```python
from build123d import *

# Parameters (mm, degrees)
SKETCH1_R                    = 11025
BOSS_EXTRUDE1_DEPTH          = 5000
BOSS_EXTRUDE2_DEPTH          = 8000
SKETCH4_R                    = 3000
CUT_EXTRUDE2_DEPTH           = 3000
SKETCH5_R                    = 1500
CUT_EXTRUDE3_DEPTH           = 3000
SKETCH6_R                    = 3000
CUT_EXTRUDE4_DEPTH           = 3000
SKETCH3_R                    = 2900
CUT_EXTRUDE1_DEPTH           = 12018
SCALE6_SCALE                 = 0.001
CORTAR_EXTRUIR1_DEPTH        = 10
CORTAR_EXTRUIR1_DEPTH_BACK   = 10
CROQUIS1_R                   = 12.5
CROQUIS2_W                   = 9
CROQUIS2_H                   = 0.876479878
CORTAR_EXTRUIR2_DEPTH        = 8
CROQUIS4_R                   = 2.9
CROQUIS4_R_2                 = 2.4
SALIENTE_EXTRUIR2_DEPTH      = 8.611616332
CROQUIS5_R                   = 3.5
CORTAR_EXTRUIR3_DEPTH        = 3
CROQUIS6_R                   = 1.591781054
CROQUIS6_R_2                 = 3
CROQUIS6_R_3                 = 1.5
CROQUIS6_R_4                 = 12.5
SALIENTE_EXTRUIR3_DEPTH      = 1
REDONDEO1_R                  = 2.5
TALADRO_DE_MARGEN_PARA_M51_D = 5.5
SALIENTE_EXTRUIR4_DEPTH      = 7
REDONDEO2_SIZE               = 2.5
REDONDEO2_SIZE_2             = 7.5


with BuildPart() as part:
    # Sketch1 → Boss-Extrude1 (new body)
    with BuildSketch(Plane.XY):
        Polygon((-21150, 17212.99935917), (-17091.781053823, 21271.218305346), (17091.781053823, 21271.218305346), (21150, 17212.99935917), (21150, -16970.562748477), (17091.781053823, -21028.781694654), (-17091.781053823, -21028.781694654), (-21150, -16970.562748477), align=None)
        with Locations((0, 121.218305346)):
            Circle(SKETCH1_R, mode=Mode.SUBTRACT)
    extrude(amount=BOSS_EXTRUDE1_DEPTH)

    # Sketch2 → Boss-Extrude2 (add)
    with BuildSketch(Plane.XY.offset(5000)):
        Polygon((0, -11028.781694654), (4500, -11028.781694654), (4500, -21028.781694654), (-4500, -21028.781694654), (-4500, -11028.781694654), align=None)
    extrude(amount=BOSS_EXTRUDE2_DEPTH)

    # Sketch4 → Cut-Extrude2 (cut)
    with BuildSketch(Plane.XY.offset(5000)):
        with Locations((-15500, 15500)):
            Circle(SKETCH4_R)
        with Locations((15500, 15500)):
            Circle(SKETCH4_R)
        with Locations((15500, -15500)):
            Circle(SKETCH4_R)
        with Locations((-15500, -15500)):
            Circle(SKETCH4_R)
    extrude(amount=-CUT_EXTRUDE2_DEPTH, mode=Mode.SUBTRACT)

    # Sketch5 → Cut-Extrude3 (cut)
    with BuildSketch(Plane.XY.offset(2000)):
        with Locations((-15500, 15500)):
            Circle(SKETCH5_R)
        with Locations((15500, -15500)):
            Circle(SKETCH5_R)
    extrude(amount=-CUT_EXTRUDE3_DEPTH, mode=Mode.SUBTRACT)

    # Sketch6 → Cut-Extrude4 (cut)
    with BuildSketch(Plane.XY.offset(2000)):
        with Locations((15500, 15500)):
            Circle(SKETCH6_R)
        with Locations((-15500, -15500)):
            Circle(SKETCH6_R)
    extrude(amount=-CUT_EXTRUDE4_DEPTH, mode=Mode.SUBTRACT)

    # Sketch3 → Cut-Extrude1 (cut)
    with BuildSketch(Plane.XZ.offset(21028.781694654)):
        with Locations(Location((0, 9000, 0), (0, 0, 270))):
            Circle(SKETCH3_R)
    extrude(amount=-CUT_EXTRUDE1_DEPTH, mode=Mode.SUBTRACT)


with BuildPart() as part_1:
    # Scale6: scaled about (0, -945.258123271, 2914.075668663)
    add(part.part.scale(SCALE6_SCALE).moved(Location((0, -944.312865148, 2911.161592994))))

    # Croquis1 → Cortar-Extruir1 (cut, two sides: drawn at the far end of the back side and taken through both)
    with BuildSketch(Plane.XY.offset(2916.161592994).offset(-CORTAR_EXTRUIR1_DEPTH_BACK)):
        with Locations(Location((0, -944.191646843, 0), (0, 0, 248.899803976))):
            Circle(CROQUIS1_R)
    extrude(amount=CORTAR_EXTRUIR1_DEPTH + CORTAR_EXTRUIR1_DEPTH_BACK, mode=Mode.SUBTRACT)

    # Croquis2 → Cortar-Extruir2 (cut)
    with BuildSketch(Plane.XY.offset(2924.161592994)):
        with Locations((0, -956.291790571)):
            Rectangle(CROQUIS2_W, CROQUIS2_H)
    extrude(amount=-CORTAR_EXTRUIR2_DEPTH, mode=Mode.SUBTRACT)

    # Croquis4 → Saliente-Extruir2 (add)
    with BuildSketch(Plane.XZ.offset(965.341646843)):
        with Locations((0, 2920.161592994)):
            Circle(CROQUIS4_R)
        with Locations(Location((0, 2920.161592994, 0), (0, 0, 270))):
            Circle(CROQUIS4_R_2, mode=Mode.SUBTRACT)
    extrude(amount=-SALIENTE_EXTRUIR2_DEPTH)

    # Croquis5 → Cortar-Extruir3 (cut)
    with BuildSketch(Plane.XY.offset(2916.161592994)):
        with Locations((-15.5, -928.812865148)):
            Circle(CROQUIS5_R)
        with Locations((15.5, -959.812865148)):
            Circle(CROQUIS5_R)
    extrude(amount=-CORTAR_EXTRUIR3_DEPTH, mode=Mode.SUBTRACT)

    # Croquis6 → Saliente-Extruir3 (add)
    with BuildSketch(Plane(origin=(0, 0, 2911.161592994), x_dir=(-1, 0, 0), z_dir=(0, 0, -1))):
        Polygon((17.091781054, -923.041646843), (-17.091781054, -923.041646843), (-21.15, -927.099865789), (-21.15, -961.283427896), (-17.091781054, -965.341646843), (17.091781054, -965.341646843), (21.15, -961.283427896), (21.15, -927.099865789), align=None)
        with Locations((15.5, -928.812865148)):
            Circle(CROQUIS6_R, mode=Mode.SUBTRACT)
        with Locations(Location((-15.5, -928.812865148, 0), (0, 0, 180))):
            Circle(CROQUIS6_R_2, mode=Mode.SUBTRACT)
        with Locations(Location((-15.5, -959.812865148, 0), (0, 0, 180))):
            Circle(CROQUIS6_R_3, mode=Mode.SUBTRACT)
        with Locations(Location((15.5, -959.812865148, 0), (0, 0, 180))):
            Circle(CROQUIS6_R_2, mode=Mode.SUBTRACT)
        with Locations((0, -944.191646843)):
            Circle(CROQUIS6_R_4, mode=Mode.SUBTRACT)
    extrude(amount=SALIENTE_EXTRUIR3_DEPTH)

    # Redondeo1
    redondeo1_edges = [part_1.edges().sort_by_distance(p)[0] for p in [
        (4.5, -961.035838676, 2924.161592994),
        (-4.5, -961.035838676, 2924.161592994),
    ]]
    fillet(redondeo1_edges, radius=REDONDEO1_R)

    # Taladro de margen para M51 (through all)
    with Locations(Plane(origin=(0, -956.73003051, 2920.161592994), x_dir=(0, 0, 1), z_dir=(0, 1, 0))):
        with Locations((0, 0)):
            Hole(TALADRO_DE_MARGEN_PARA_M51_D / 2)

    # Croquis8 → Saliente-Extruir4 (add)
    with BuildSketch(Plane.XZ.offset(965.341646843)):
        Polygon((-2.879289322, 2912.011592994), (-5.45, 2912.011592994), (-5.45, 2913.290882316), (-2.529289322, 2916.211592994), (2.429289322, 2916.211592994), (5.35, 2913.290882316), (5.35, 2912.011592994), (2.879289322, 2912.011592994), (2.879289322, 2910.161592994), (-2.879289322, 2910.161592994), align=None)
    extrude(amount=SALIENTE_EXTRUIR4_DEPTH)

    # Redondeo2
    # an asymmetric fillet: 7.5, 2.5 mm, written as the material it adds along each edge
    with BuildSketch(Plane(origin=(4.5, -956.73003051, 2916.161592994), x_dir=(0, 0, 1), z_dir=(0, -1, 0))) as redondeo2_piece_1:
        with BuildLine():
            Bezier((REDONDEO2_SIZE, 0), (0, 0), (0, -REDONDEO2_SIZE_2), weights=[1, 0.707106781, 1])
            Line((0, -REDONDEO2_SIZE_2), (0, 0))
            Line((0, 0), (REDONDEO2_SIZE, 0))
        make_face()
    extrude(amount=8.611616332)
    with BuildSketch(Plane(origin=(-4.5, -965.341646842, 2916.161592994), x_dir=(-1, 0, 0), z_dir=(0, 1, 0))) as redondeo2_piece_2:
        with BuildLine():
            Bezier((REDONDEO2_SIZE_2, 0), (0, 0), (0, REDONDEO2_SIZE), weights=[1, 0.707106781, 1])
            Line((0, REDONDEO2_SIZE), (0, 0))
            Line((0, 0), (REDONDEO2_SIZE_2, 0))
        make_face()
    extrude(amount=8.611616332)


solid = part_1.part
```
Can you work these out from the model? Positions are in its coordinate system, mm. A direction names the side the tool comes from. Round coordinates to 2 decimals unless told otherwise and drop trailing zeros. Loops run counter-clockwise (first coordinate to the right, second up) from the corner with the lowest first, then second, coordinate; pieces in that order, holes last. Notation, with made-up numbers: (45.5, 48) -> (59.5, 48) arc R12 ccw to (59.5, 61) -> close; hole circle Ø4 at (-27.75, 56.5). An arc over 180 degrees is marked (long way). Answer in a Markdown table with one row per item.
Item 1: Suppose I cut it at A-A, the plane x = 15.5. List the corners of the cut face in (y, z) for me, plus the area to 3 significant figures.
Answer block:
| item | result |
|---|---|
| outline | (-965.34, 2910.16) -> (-961.31, 2910.16) -> (-961.31, 2913.16) -> (-963.31, 2913.16) -> (-963.31, 2916.16) -> (-965.34, 2916.16) -> close; (-958.31, 2910.16) -> (-931.81, 2910.16) -> (-931.81, 2916.16) -> (-956.31, 2916.16) -> (-956.31, 2913.16) -> (-958.31, 2913.16) -> close; (-925.81, 2910.16) -> (-923.04, 2910.16) -> (-923.04, 2916.16) -> (-925.81, 2916.16) -> close |
| area | 188 mm² |
Item 2: Suppose I cut it at D-D, the plane x = -15.5. List the corners of the cut face in (y, z) for me.
Answer block:
| item | result |
|---|---|
| outline | (-965.34, 2910.16) -> (-962.81, 2910.16) -> (-962.81, 2916.16) -> (-965.34, 2916.16) -> close; (-956.81, 2910.16) -> (-930.4, 2910.16) -> (-930.4, 2911.16) -> (-930.31, 2911.16) -> (-930.31, 2913.16) -> (-932.31, 2913.16) -> (-932.31, 2916.16) -> (-956.81, 2916.16) -> close; (-927.31, 2911.16) -> (-927.22, 2911.16) -> (-927.22, 2910.16) -> (-923.04, 2910.16) -> (-923.04, 2916.16) -> (-925.31, 2916.16) -> (-925.31, 2913.16) -> (-927.31, 2913.16) -> close |
Item 3: Suppose I cut it at C-C, the plane z = 2920.25. List the corners of the cut face in (x, y) for me, plus the area to 3 significant figures.
Answer block:
| item | result |
|---|---|
| outline | (-4.5, -965.34) -> (-2.75, -965.34) -> (-2.75, -956.73) -> (-4.5, -956.73) -> close; (2.75, -965.34) -> (4.5, -965.34) -> (4.5, -956.73) -> (2.75, -956.73) -> close |
| area | 30.2 mm² |
Item 4: Suppose I cut it at B-B, the plane y = -946. List the corners of the cut face in (x, z) for me.
Answer block:
| item | result |
|---|---|
| outline | (-21.15, 2910.16) -> (-12.37, 2910.16) -> (-12.37, 2916.16) -> (-21.15, 2916.16) -> close; (12.37, 2910.16) -> (21.15, 2910.16) -> (21.15, 2916.16) -> (12.37, 2916.16) -> close |
Item 5: Will these pins go through, and if not, where does the flat tip stop? P1, Ø3.5, axis at x = -15.5, y = -928.5, coming from the -Z side; P2, Ø2, axis at y = -969, z = 2911.5, coming from the -X side; P3, Ø0.6, axis at y = -970, z = 2912.5, coming from the +X side; P4, Ø5, axis at x = 15.5, y = -928.81, coming from the +Z side.
Answer block:
| item | result |
|---|---|
| P1 | z = 2910.16 |
| P2 | x = -5.45 |
| P3 | x = 5.35 |
| P4 | through |
Item 6: On a 3-axis mill with a long thin cutter (end or side, diameter ignored), from which of +Z, -Z, +X, -X, +Y, -Y can I reach the whole of each face in a straight line? I mean faces 4 (the cylindrical face through (-16.235, -930.225, 2910.669)), 5 (the flat face through (3.87, -968.79, 2914.77)), 6 (the flat face through (-5.45, -969, 2913)). Say none if no direction works.
Answer block:
| item | result |
|---|---|
| face 4 | -Z |
| face 5 | +Z, +X, -Y |
| face 6 | +Z, -Z, -X, -Y |
Item 7: We'd pull the mould along Y, two halves only. Please class faces 1 (the flat face through (17, -961, 2913.162)), 2 (the flat face through (19.09, -925.04, 2913.2)), 3 (the flat face through (0, -930, 2916.162)): released by +Y, released by -Y, zero draft, split by the parting line, or undercut.
Answer block:
| item | result |
|---|---|
| face 1 | undercut |
| face 2 | released by +Y |
| face 3 | zero draft |
Item 8: If I drill on probe 1 along Y at (x, z) = (-15.5, 2910.6); probe 2 along Y at (x, z) = (-15.5, 2914.4); probe 3 along Y at (x, z) = (0.5, 2915.25), over which ranges is the centre line in solid material (lowest first)?
Answer block:
| item | result |
|---|---|
| probe 1 | -965.34 to -962.81, -956.81 to -930.4, -927.22 to -923.04 |
| probe 2 | -965.34 to -962.81, -956.81 to -932.31, -925.31 to -923.04 |
| probe 3 | -972.34 to -956.68, -931.7 to -923.04 |
